Could you check a few things on this model? Use its own coordinates, in mm. A direction names the side the tool comes from. Give positions to 0.01 mm unless a question says otherwise; leave off trailing zeros. Use a Markdown table: item, result. Add a question column.
Autodesk Inventor part; units mm, degrees
ref_plane "YZ Plane" through (0, 0, 0) normal (1, 0, 0) x (0, 1, 0)
ref_plane "XZ Plane" through (0, 0, 0) normal (0, 1, 0) x (-1, 0, 0)
ref_plane "XY Plane" through (0, 0, 0) normal (0, 0, 1) x (1, 0, 0)
sketch "Sketch1" plane through (0, 0, 0) normal (0, 1, 0) x (-1, 0, 0)
  line L0 (0, 0) -> (150, 0)
  line L1 (150, 0) -> (150, -140)
  line L2 (150, -140) -> (0, -140)
  line L3 (0, -140) -> (0, 0)
  dimension "d0" = 140
  dimension "d2" = 150
extrude "Extrusion1" add sketch "Sketch1" along normal blind 86
sketch "Sketch2" plane through (-150, 0, 0) normal (0, 0, 1) x (1, 0, 0)
  line L0 (150, 0) -> (0, 0)
  line L1 (0, 0) -> (6, 0)
  line L2 (6, 0) -> (6, 16)
  line L3 (6, 16) -> (6, 80)
  line L4 (6, 80) -> (144, 80)
  line L5 (0, 0) -> (0, 86)
  line L6 (6, 80) -> (144, 80) construction
  circle A0 centre (6, 16) radius 1.75
  line L7 (120, 0) -> (120, 6)
  circle A1 centre (120, 6) radius 1.75
  circle A2 centre (6, 80) radius 1.75
  circle A3 centre (144, 80) radius 1.75
  dimension "d5" = 6
  dimension "d6" = 16
  dimension "d7" = 64
  dimension "d8" = 138
  dimension "d9" = 360
  dimension "d10" = 6
  dimension "d11" = 114
  dimension "d12" = 74
  dimension "d13" = 3.5
  dimension "d14" = 3.5
  dimension "d15" = 3.5
  dimension "d16" = 3.5
extrude "Extrusion2" cut sketch "Sketch2" against normal blind 4.7625
sketch "Sketch3" plane through (0, 86, 0) normal (0, 1, 0) x (1, 0, 0)
  line L0 (-150, 140) -> (-150, 0)
  line L1 (-150, 140) -> (-75, 140)
  line L2 (-75, 140) -> (-75, 70)
  line L3 (-75, 70) -> (-150, 70)
  line L4 (-150, 70) -> (-150, 140)
  line L5 (0, 0) -> (0, 140)
  line L6 (-150, 140) -> (0, 140)
  line L7 (0, 140) -> (0, 0)
  line L8 (0, 0) -> (-150, 0)
  line L9 (-150, 0) -> (-150, 140)
  circle A0 centre (-75, 70) radius 61.5476
  dimension "d19" = 70
  dimension "d20" = 140
  dimension "d21" = 150
  dimension "d22" = 75
extrude "Extrusion3" cut sketch "Sketch3" against normal blind 0.01 contours A0 L2 L3 | L3 L2 A0
equation "\"d14\" = d13"
equation "\"d15\" = d13"
equation "\"d16\" = d13"
equation "\"d19\" = 0.5 * d20"
equation "\"d22\" = 0.5 * d21"
properties part number "PSU"
1) Please list where these lines run through material, in increasing order: line 1 (Y direction, x = -144, z = -1.45); line 2 (X direction, y = 80, z = -1); line 3 (X direction, y = 16, z = -1.15). Write a range as from..to.
2) For faces 1 (the face through (-6, 80, -4.762)), 2 (the face through (-76, 85.99, -71)), which set-ups out of +Z, -Z, +X, -X, +Y, -Y let a thin tool reach every point of the face, with its end or its side?
3) For pin 1 (3 mm diameter, centred on x = -84.5, z = -70.5, fed in from +Y); pin 2 (3 mm diameter, centred on x = -144, y = 16, fed in from +Z), each with a flat end and sliding along its axis, tell me the tip position at first contact or that it passes through.
Values found:
| question | item | result |
|---|---|---|
| 1 | line 1 | y = 0..14.25, 17.75..78.25, 81.75..86 |
| 1 | line 2 | x = -150..-145.75, -142.25..-7.75, -4.25..0 |
| 1 | line 3 | x = -150..-145.75, -142.25..0 |
| 2 | face 1 | +Z |
| 2 | face 2 | +Z, -Z, +X, -X, +Y |
| 3 | pin 1 | stops at y = 85.99 |
| 3 | pin 2 | stops at z = -4.76 |
